Here's how the part is built. I have some questions about the finished solid (model axes, mm). Face numbers are marked on the shaded views. A direction names the side the tool comes from. Round coordinates to 2 decimals unless told otherwise and drop trailing zeros. Order: outer loops, then holes, each group sorted by start corner. A loop starts at its lowest first (then second) coordinate and runs counter-clockwise, first axis right, second up. Notation, with made-up numbers: (23.25, -3) -> (53.25, -3) arc R20 cw to (53.25, 4) -> close; hole circle Ø3 at (81.25, 6.25). An arc over 180 degrees is marked (long way). Use a Markdown table: item, result. Add a question column.
(1) I'm going to push flat-ended pins straight in: P1, Ø12, axis at y = -23, z = -3.5, coming from the -X side; P2, Ø4, axis at y = -31.5, z = 0.5, coming from the -X side; P3, Ø2, axis at x = -32, z = 21.945, coming from the -Y side; P4, Ø3, axis at y = -31, z = 10.5, coming from the +X side. Where does each tip first touch, or does it pass through?
(2) If I drill on probe 1 along Z at (x, y) = (-32, -1.2) (3 decimals); probe 2 along Y at (x, z) = (-37, 27); probe 3 along X at (y, z) = (-20.5, -17), over which ranges is the centre line in solid material (lowest first)?
(3) I want a section at C-C, the plane z = -26. Please give me the cut outline in (x, y), then the cut area to 3 significant figures.
(4) I want a section at A-A, the plane x = -32. Please give me the cut outline in (y, z) (3 decimals).
(5) I want a section at B-B, the plane y = -29. Please give me the cut outline in (x, z) (3 decimals).
(6) On a 3-axis mill with a long thin cutter (end or side, diameter ignored), from which of +Z, -Z, +X, -X, +Y, -Y can I reach the whole of each face in a straight line? I mean the marked faces 1 and 2. Say none if no direction works.
(7) I want a section at D-D, the plane x = -81.5. Please give me the cut outline in (y, z) (1 decimal).
(8) Thinking about a two-plate mould opening in X: for the marked faces 3, 4 and 5, which applies, pulls with the +X half, pulls with the -X half, needs draft (parallel to the pull), parting line crosses it, or undercut?
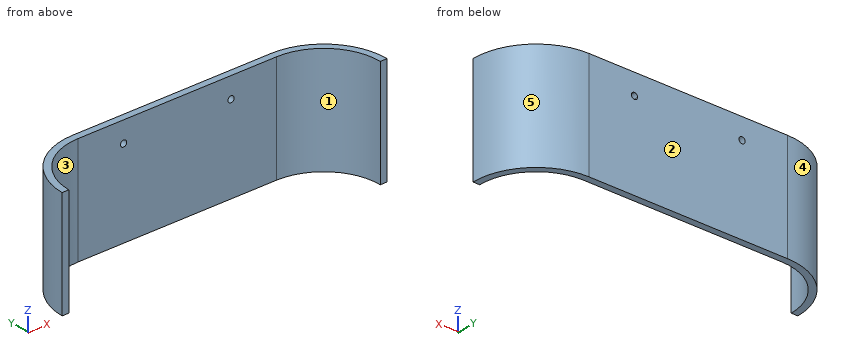
from build123d import *

# Parameters (mm, degrees)
F0_W     = 118.1
F0_H     = 60.85
F1_DEPTH = 2.5
F4_DEPTH = 32.925
F5_DEPTH = 30.425
F6_DEPTH = 2.5
F7_DEPTH = 1.5
F9_DEPTH = 25


# Not quite as in the source:
# - a feature of the source that left no trace in its solid (it failed there, or was rolled back) is left out
# - a pattern or mirror of a feature is missing from the dataset's text; its kind, count and spacing are read off the source's solid


with BuildPart() as f1:
    # F0 (on Front) → F1 (new body)
    with BuildSketch(Plane.XZ):
        Rectangle(F0_W, F0_H)
    extrude(amount=F1_DEPTH)

    # F1_copies: F1 across plane


with BuildPart() as f1_1:
    add(f1.part)
    add(f1.part.mirror(Plane.ZX.offset(-0.5)))

    # F3 (on Top) → F4 (join)
    with BuildSketch(Plane.XY):
        with BuildLine():
            ThreePointArc((-92.7, -36.15), (-82.8441431869, -12.3558568131), (-59.05, -2.5))
            Line((-59.05, -2.5), (-59.05, 0))
            Line((-59.05, 0), (-59.05, 1.5))
            ThreePointArc((-59.05, 1.5), (-85.6725703117, -9.5274296883), (-96.7, -36.15))
            Line((-96.7, -36.15), (-95.2, -36.15))
            Line((-95.2, -36.15), (-92.7, -36.15))
        make_face()
        with BuildLine():
            ThreePointArc((59.05, -2.5), (82.8441431869, -12.3558568131), (92.7, -36.15))
            Line((92.7, -36.15), (95.2, -36.15))
            Line((95.2, -36.15), (96.7, -36.15))
            ThreePointArc((96.7, -36.15), (85.6725703117, -9.5274296883), (59.05, 1.5))
            Line((59.05, 1.5), (59.05, 0))
            Line((59.05, 0), (59.05, -2.5))
        make_face()
    extrude(amount=F4_DEPTH)

    # F3 (on Top) → F5 (join)
    with BuildSketch(Plane.XY):
        with BuildLine():
            ThreePointArc((-92.7, -36.15), (-82.8441431869, -12.3558568131), (-59.05, -2.5))
            Line((-59.05, -2.5), (-59.05, 0))
            Line((-59.05, 0), (-59.05, 1.5))
            ThreePointArc((-59.05, 1.5), (-85.6725703117, -9.5274296883), (-96.7, -36.15))
            Line((-96.7, -36.15), (-95.2, -36.15))
            Line((-95.2, -36.15), (-92.7, -36.15))
        make_face()
        with BuildLine():
            ThreePointArc((59.05, -2.5), (82.8441431869, -12.3558568131), (92.7, -36.15))
            Line((92.7, -36.15), (95.2, -36.15))
            Line((95.2, -36.15), (96.7, -36.15))
            ThreePointArc((96.7, -36.15), (85.6725703117, -9.5274296883), (59.05, 1.5))
            Line((59.05, 1.5), (59.05, 0))
            Line((59.05, 0), (59.05, -2.5))
        make_face()
    extrude(amount=-F5_DEPTH)

    # F6 (add): a face of the model
    f6_faces = [f1_1.faces().sort_by_distance(p)[0] for p in [
        (0, -0.5, 30.425),
    ]]
    extrude(f6_faces, amount=F6_DEPTH)

    # F7 (add): a face of the model
    f7_faces = [f1_1.faces().sort_by_distance(p)[0] for p in [
        (84.2373603721, -10.9626396279, 32.925),
    ]]
    extrude(f7_faces, amount=F7_DEPTH)

    # F8 (on face) → F9 (cut)
    with BuildSketch(Plane(origin=(0, 1.5, 0), x_dir=(-1, 0, 0), z_dir=(0, 1, 0))):
        with BuildLine():
            ThreePointArc((33.85, 21.945), (32, 23.795), (30.15, 21.945))
            ThreePointArc((30.15, 21.945), (32, 20.095), (33.85, 21.945))
        make_face()
        with BuildLine():
            ThreePointArc((-32, 23.795), (-33.3081475452, 20.6368524548), (-30.15, 21.945))
            ThreePointArc((-30.15, 21.945), (-30.6918524548, 23.2531475452), (-32, 23.795))
        make_face()
    extrude(amount=-F9_DEPTH, mode=Mode.SUBTRACT)


solid = f1_1.part
Taken from the geometry:
| question | item | result |
|---|---|---|
| 1 | P1 | stops at x = -96.01 |
| 1 | P2 | stops at x = -96.61 |
| 1 | P3 | passes through |
| 1 | P4 | stops at x = 96.52 |
| 2 | probe 1 | z = -30.425 to 20.095, 23.795 to 34.425 |
| 2 | probe 2 | y = -2.5 to 1.5 |
| 2 | probe 3 | x = -93.29 to -88.84, 88.84 to 93.29 |
| 3 | outline | (-96.7, -36.15) -> (-92.7, -36.15) arc R33.65 cw to (-59.05, -2.5) -> (59.05, -2.5) arc R33.65 cw to (92.7, -36.15) -> (96.7, -36.15) arc R37.65 ccw to (59.05, 1.5) -> (-59.05, 1.5) arc R37.65 ccw to start |
| 3 | area | 920 mm2 |
| 4 | outline | (-2.5, -30.425) -> (1.5, -30.425) -> (1.5, 20.095) -> (-2.5, 20.095) -> close; (-2.5, 23.795) -> (1.5, 23.795) -> (1.5, 34.425) -> (-2.5, 34.425) -> close |
| 5 | outline | (-96.015, -30.425) -> (-91.932, -30.425) -> (-91.932, 34.425) -> (-96.015, 34.425) -> close; (91.932, -30.425) -> (96.015, -30.425) -> (96.015, 34.425) -> (91.932, 34.425) -> close |
| 6 | face 1 | +Z, -Z, -Y |
| 6 | face 2 | +Z, -Z, +X, -X, +Y |
| 7 | outline | (-11.1, -30.4) -> (-5.9, -30.4) -> (-5.9, 34.4) -> (-11.1, 34.4) -> close |
| 8 | face 3 | undercut |
| 8 | face 4 | pulls with the -X half |
| 8 | face 5 | pulls with the +X half |
